Study the drawing (mm; zero at the part's minimum x, y, z) and answer. Give positions to 0.01 mm unless a question says otherwise; leave off trailing zeros. Order: outer loops, then holes, each group sorted by start corner. A loop starts at its lowest first (then second) coordinate and runs counter-clockwise, first axis right, second up.
Item 1: A cutting plane is placed at B-B (x = 17.5). Write down the section's boundary in (y, z).
Item 2: A cutting plane is placed at C-C (x = 284). Write down the section's boundary in (y, z), plus the area to 3 significant figures.
Item 3: Find the intervals of material crossed by line 1 along X through (y, z) = (5, 17.5); line 2 along Z through (x, y) = (297.5, 1.5); line 3 along X through (y, z) = (5, 15) (1 decimal), in increasing order.
Item 4: Given pin 1 Ø5 at (x, z) = (237, 25) entering from -Y; pin 2 Ø3 at (x, y) = (212, 2.5) entering from -Z; pin 3 Ø1 at (y, z) = (1.5, 31.5) entering from -X (1 decimal); pin 4 Ø2 at (x, y) = (162.5, 3) entering from +Z, each flat-ended and moving along its own axis, determine where each tip first touches the part or whether it passes through.
Item 5: A cutting plane is placed at A-A (y = 3.5). State how many separate pieces and enclosed holes the cut face has, plus the area to 3 significant figures.
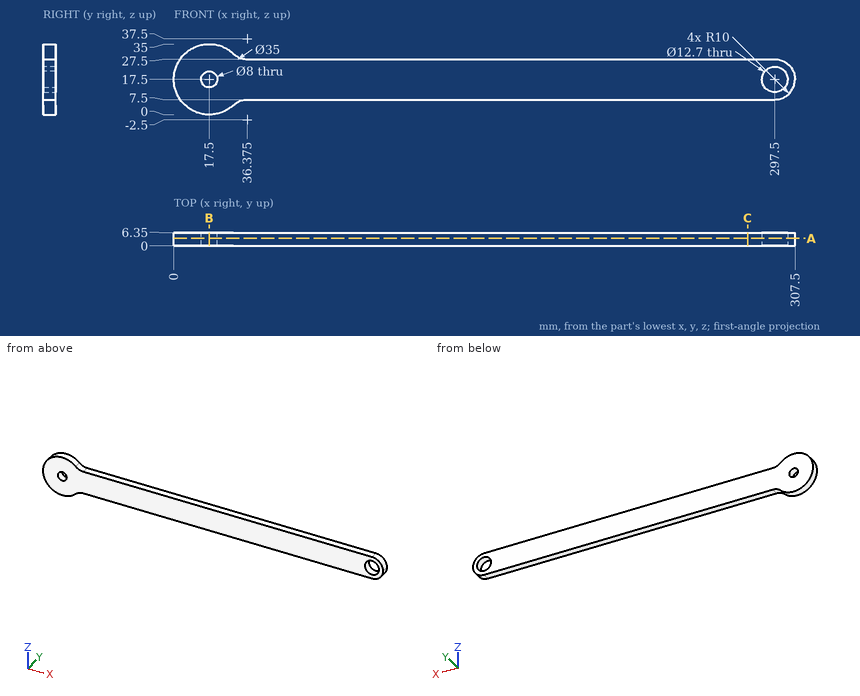
Response values:
1. outline: (0, 0) - (6.35, 0) - (6.35, 13.5) - (0, 13.5) - close; (0, 21.5) - (6.35, 21.5) - (6.35, 35) - (0, 35) - close
2. outline: (0, 7.5) - (6.35, 7.5) - (6.35, 27.5) - (0, 27.5) - close
2. area: 127 mm2
3. line 1: x = 0 to 13.5, 21.5 to 291.15, 303.85 to 307.5
3. line 2: z = 7.5 to 11.15, 23.85 to 27.5
3. line 3: x = 0.2 to 14.4, 20.6 to 291.7, 303.3 to 307.2
4. pin 1: stops at y = 0
4. pin 2: stops at z = 7.5
4. pin 3: stops at x = 6.4
4. pin 4: stops at z = 27.5
5. separate pieces: 1
5. enclosed holes: 2
5. area: 6,220 mm2
